```python
from build123d import *

# Parameters (mm, degrees)
SKETCH_1_R          = 1.45
EXTRUDE_1_DEPTH     = 1.6
CUT_EXTRUDE_1_DEPTH = 1.6
CUT_EXTRUDE_2_DEPTH = 1.6


with BuildPart() as part:
    # 草图1 → 凸台-拉伸1 (new body)
    with BuildSketch(Plane.XY):
        with BuildLine():
            Line((-30, 32.8), (30, 32.8))
            ThreePointArc((30, 32.8), (31.979898987, 31.979898987), (32.8, 30))
            Line((32.8, 30), (32.8, -30))
            ThreePointArc((32.8, -30), (31.979898987, -31.979898987), (30, -32.8))
            Line((30, -32.8), (-30, -32.8))
            ThreePointArc((-30, -32.8), (-31.979898987, -31.979898987), (-32.8, -30))
            Line((-32.8, -30), (-32.8, 30))
            ThreePointArc((-32.8, 30), (-31.979898987, 31.979898987), (-30, 32.8))
        make_face()
        with Locations((-30, 30)):
            Circle(SKETCH_1_R, mode=Mode.SUBTRACT)
        with Locations((30, 30)):
            Circle(SKETCH_1_R, mode=Mode.SUBTRACT)
        with Locations((-30, -30)):
            Circle(SKETCH_1_R, mode=Mode.SUBTRACT)
        with Locations((30, -30)):
            Circle(SKETCH_1_R, mode=Mode.SUBTRACT)
    extrude(amount=EXTRUDE_1_DEPTH)

    # 草图2 → 切除-拉伸1 (cut)
    with BuildSketch(Plane.XY.offset(1.6)):
        Polygon((-25.8, 29.06), (-19.8, 29.06), (-19.8, 28.06), (-22.3, 28.06), (-22.3, 23.06), (-23.3, 23.06), (-23.3, 28.06), (-25.8, 28.06), align=None)
    extrude(amount=-CUT_EXTRUDE_1_DEPTH, mode=Mode.SUBTRACT)

    # 草图3 → 切除-拉伸2 (cut)
    with BuildSketch(Plane.XY.offset(1.6)):
        Polygon((25.3, -1), (27.8, -1), (27.8, 0), (21.8, 0), (21.8, -1), (24.3, -1), (24.3, -6), (25.3, -6), align=None)
    extrude(amount=-CUT_EXTRUDE_2_DEPTH, mode=Mode.SUBTRACT)


solid = part.part
```
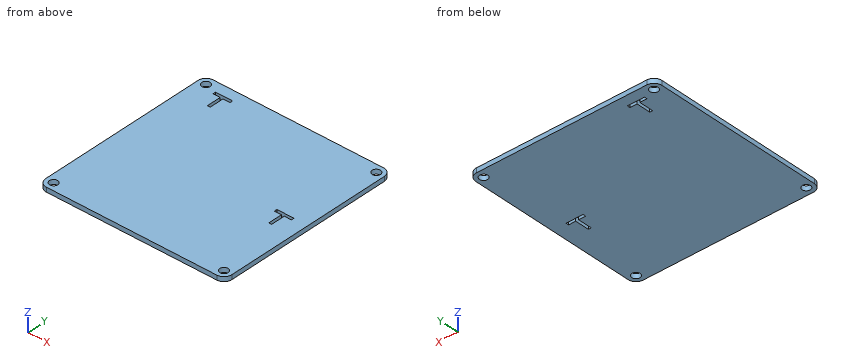
Build history of the part. All positions in model axes, mm. Coordinates: 2 decimals unless noted, no trailing zeros. Order: outer loops, then holes, each group sorted by start corner. A loop starts at its lowest first (then second) coordinate and runs counter-clockwise, first axis right, second up. Notation, with made-up numbers: M 82.25,-19.75 L 131.25,-19.75 A15 ccw 131.25,-3.75 Z; hole C -32,57.25 d3. An arc over 180 degrees is marked long. One line per question, with ' | ' between items. Start each with the question number.
1. Cut at A-A (y = 27). Write the cut outline in (x, z), plus the area to 3 significant figures.
2. Flat gauge pins, fed straight in: P1, Ø4, axis at x = 30, y = -30, coming from the +Z side; P2, Ø2.5, axis at x = -30, y = -30, coming from the +Z side. Where does each tip first touch, or does it go through?
3. Wall check: line 1 along Y through (x, z) = (-30, 0.65); line 2 along X through (y, z) = (27, 0.65). Give the ranges that are in metal, low to high. Write a range as [from, to].
The answers:
1) outline: M -32.8,0 L -23.3,0 L -23.3,1.6 L -32.8,1.6 Z; M -22.3,0 L 32.8,0 L 32.8,1.6 L -22.3,1.6 Z | area: 103 mm2
2) P1: stops at z = 1.6 | P2: passes through
3) line 1: y = [-32.8, -31.45], [-28.55, 28.55], [31.45, 32.8] | line 2: x = [-32.8, -23.3], [-22.3, 32.8]
